from build123d import *

# Parameters (mm, degrees)
F0_W     = 13.0048
F0_H     = 6.6548
F1_DEPTH = 10.668
F2_R     = 19.05
F3_DEPTH = 15.24
F4_R     = 2.54
F5_R     = 14.859
F6_DEPTH = 5.334
F7_R     = 1.651
F8_DEPTH = 21.59


with BuildPart() as f1:
    # F0 (on Top) → F1 (new body)
    with BuildSketch(Plane.XY):
        Rectangle(F0_W, F0_H)
    extrude(amount=F1_DEPTH)

    # F2 (on face) → F3 (join)
    with BuildSketch(Plane(origin=(0, 0, 0), x_dir=(1, 0, 0), z_dir=(0, 0, -1))):
        Circle(F2_R)
    extrude(amount=F3_DEPTH)

    # F4
    f4_edges = [f1.edges().sort_by_distance(p)[0] for p in [
        (-19.05, 0, 0),
    ]]
    fillet(f4_edges, radius=F4_R)

    # F5 (on face) → F6 (cut)
    with BuildSketch(Plane(origin=(0, 0, -15.24), x_dir=(1, 0, 0), z_dir=(0, 0, -1))):
        Circle(F5_R)
    extrude(amount=-F6_DEPTH, mode=Mode.SUBTRACT)

    # F7 (on face) → F8 (cut)
    with BuildSketch(Plane(origin=(0, 0, -9.906), x_dir=(1, 0, 0), z_dir=(0, 0, -1))):
        Circle(F7_R)
    extrude(amount=-F8_DEPTH, mode=Mode.SUBTRACT)


solid = f1.part
The listing builds one solid part. Answer for the finished solid, in the listing's coordinates (mm). A direction names the side the tool comes from. Round coordinates to 2 decimals unless told otherwise and drop trailing zeros. Write each loop counter-clockwise with the first axis right and the second up, starting at its lowest first coordinate (ties: lowest second). Pieces come first, ordered by that corner, then holes. Notation, with made-up numbers: (82.25, 84) - (104.25, 84) arc R30 ccw to (104.25, 112) - close; hole circle Ø3 at (63, 57). An arc over 180 degrees is marked (long way). Use a Markdown table: item, result. Add a question column.
1. The part is cut by section B-B (x = 0). Write down the section's boundary in (y, z), and give its area (3 significant figures).
2. The part is cut by section A-A (y = 0). Write down the section's boundary in (x, z), and give its area (3 significant figures).
3. The part is cut by section C-C (z = -5.5). Write down the section's boundary in (x, y), and give its area (3 significant figures).
4. Consider line 1 (X direction, y = 0, z = -13.65); line 2 (X direction, y = 0, z = -3); line 3 (Y direction, x = 0, z = 1.75). Determine where each line is inside the solid, lowest interval first.
5. For a pull along X with two mould halves and no side action, classify faces 1 (the face through (6.502, 0, 5)), 2 (the face through (-15.12, 11.59, -8.8)), 3 (the face through (0, 3.327, 5)), 4 (the face through (1.525, 0.632, 0.237)) as +X half, -X half, draft (parallel to the pull), parting line (faces both ways), or undercut.
6. A tool of negligible diameter and unlimited length cuts with its end or side. For faces 5 (the face through (0, -3.327, 5)), 6 (the face through (-10, 11.2, -15.24)), 7 (the face through (0, 3, -9.906)), 8 (the face through (-6.502, 0, 5)), from which of +Z, -Z, +X, -X, +Y, -Y can it reach the whole face along a straight path? Write none if from no direction.
7. Flat-ended cylindrical pins translate along their axes: P1, Ø8, axis at x = 4.5, z = -4.5, coming from the +Y side; P2, Ø2, axis at y = 1, z = 8, coming from the -X side; P3, Ø5.5, axis at y = 1, z = 7.5, coming from the +X side. Find the tip coordinate at first contact, or state that the pin passes through.
Reported:
| question | item | result |
|---|---|---|
| 1 | outline | (-19.05, -15.24) - (-14.86, -15.24) - (-14.86, -9.91) - (-1.65, -9.91) - (-1.65, 10.67) - (-3.33, 10.67) - (-3.33, 0) - (-16.51, 0) arc R2.54 ccw to (-19.05, -2.54) - close; (1.65, -9.91) - (14.86, -9.91) - (14.86, -15.24) - (19.05, -15.24) - (19.05, -2.54) arc R2.54 ccw to (16.51, 0) - (3.33, 0) - (3.33, 10.67) - (1.65, 10.67) - close |
| 1 | area | 422 mm^2 |
| 2 | outline | (-19.05, -15.24) - (-14.86, -15.24) - (-14.86, -9.91) - (-1.65, -9.91) - (-1.65, 10.67) - (-6.5, 10.67) - (-6.5, 0) - (-16.51, 0) arc R2.54 ccw to (-19.05, -2.54) - close; (1.65, -9.91) - (14.86, -9.91) - (14.86, -15.24) - (19.05, -15.24) - (19.05, -2.54) arc R2.54 ccw to (16.51, 0) - (6.5, 0) - (6.5, 10.67) - (1.65, 10.67) - close |
| 2 | area | 490 mm^2 |
| 3 | outline | circle Ø38.1 at (0, 0); hole circle Ø3.3 at (0, 0) |
| 3 | area | 1,130 mm^2 |
| 4 | line 1 | -19.05 to -14.86, 14.86 to 19.05 |
| 4 | line 2 | -19.05 to -1.65, 1.65 to 19.05 |
| 4 | line 3 | -3.33 to -1.65, 1.65 to 3.33 |
| 5 | face 1 | +X half |
| 5 | face 2 | parting line |
| 5 | face 3 | draft |
| 5 | face 4 | undercut |
| 6 | face 5 | +Z, +X, -X, -Y |
| 6 | face 6 | -Z, +X, -X, +Y, -Y |
| 6 | face 7 | -Z |
| 6 | face 8 | +Z, -X, +Y, -Y |
| 7 | P1 | y = 19.04 |
| 7 | P2 | x = -6.5 |
| 7 | P3 | x = 6.5 |
